```python
from build123d import *

# Parameters (mm, degrees)
F0_R     = 22.5
F1_DEPTH = 120
F3_DEPTH = 70
F4_R     = 20
F5_DEPTH = 35
F6_R     = 2.5
F7_DEPTH = 50


with BuildPart() as f1:
    # F0 (on Top) → F1 (new body)
    with BuildSketch(Plane.XY):
        Circle(F0_R)
    extrude(amount=F1_DEPTH)

    # F2 (on face) → F3 (cut)
    with BuildSketch(Plane.XY.offset(120)):
        with BuildLine():
            ThreePointArc((22.5, 0), (19.843135, 10.606602), (12.5, 18.708287))
            Line((12.5, 18.708287), (12.5, -18.708287))
            ThreePointArc((12.5, -18.708287), (19.843135, -10.606602), (22.5, 0))
        make_face()
        with BuildLine():
            Line((-12.5, -18.708287), (-12.5, 18.708287))
            ThreePointArc((-12.5, 18.708287), (-22.5, 0), (-12.5, -18.708287))
        make_face()
    extrude(amount=-F3_DEPTH, mode=Mode.SUBTRACT)

    # F4 (on Top) → F5 (cut)
    with BuildSketch(Plane.XY):
        Circle(F4_R)
    extrude(amount=F5_DEPTH, mode=Mode.SUBTRACT)

    # F6 (on Right) → F7 (cut, symmetric)
    with BuildSketch(Plane.YZ):
        with Locations((0, 100)):
            Circle(F6_R)
    extrude(amount=F7_DEPTH, both=True, mode=Mode.SUBTRACT)


solid = f1.part
```
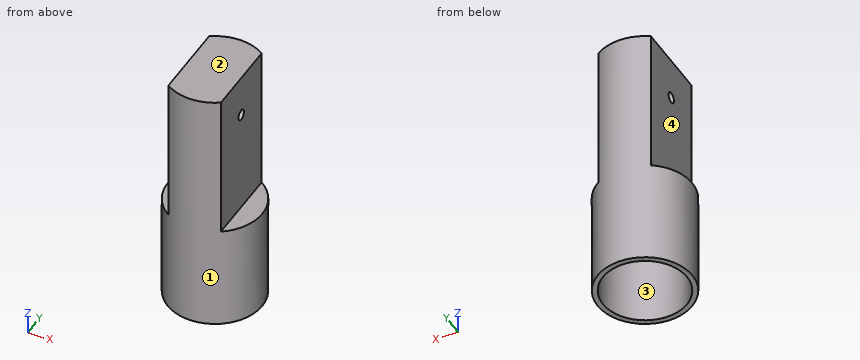
Check sheet for the modelled part. Datum: model origin and axes. Units: mm. Face numbers are marked on the shaded views. Coordinates: 2 decimals unless noted, no trailing zeros. Order: outer loops, then holes, each group sorted by start corner. A loop starts at its lowest first (then second) coordinate and runs counter-clockwise, first axis right, second up. Notation, with made-up numbers: (-3.75, -33) -> (14.25, -33) arc R12 cw to (14.25, -17) -> close; hole circle Ø1 at (-8.75, 83). An arc over 180 degrees is marked (long way). Write each question's results on one line, items separated by ' | '. Start each with the question number.
1) Draft check along X on the marked faces 1, 2, 3 and 4. Enter one of: pulls with the +X half, pulls with the -X half, needs draft (parallel to the pull), parting line crosses it, or undercut.
2) Depth check by flat-ended pin: pin 1 (1 mm diameter, centred on x = 17.5, y = 9, fed in from +Z); pin 2 (11 mm diameter, centred on y = 1, z = 76, fed in from -X); pin 3 (1.5 mm diameter, centred on x = 6, z = 61.5, fed in from +Y); pin 4 (11 mm diameter, centred on x = 15.5, y = -1, fed in from +Z). Enter the tip coordinate at first touch or a pass-through.
3) Material ranges on line 1 along Y through (x, z) = (0, 12); line 2 along Z through (x, y) = (4, 0); line 3 along Z through (x, y) = (-10, -4.5), recorded low to high.
4) Section check D-D (y = 13). Enter the section's corners in (x, z), and give its area (3 significant figures).
5) Section check A-A (z = 100). Enter the section's corners in (x, y), and give its area (3 significant figures).
6) Section check C-C (x = -4). Enter the section's corners in (y, z), and give its area (3 significant figures).
7) Section check B-B (y = 0). Enter the section's corners in (x, z), and give its area (4 significant figures).
Checked values:
1) face 1: parting line crosses it | face 2: needs draft | face 3: undercut | face 4: pulls with the -X half
2) pin 1: z = 50 | pin 2: x = -12.5 | pin 3: y = 21.88 | pin 4: z = 120
3) line 1: -22.5 to -20, 20 to 22.5 | line 2: 35 to 97.5, 102.5 to 120 | line 3: 35 to 120
4) outline: (-18.36, 0) -> (-15.2, 0) -> (-15.2, 35) -> (15.2, 35) -> (15.2, 0) -> (18.36, 0) -> (18.36, 50) -> (12.5, 50) -> (12.5, 120) -> (-12.5, 120) -> (-12.5, 50) -> (-18.36, 50) -> close | area: 2,520 mm²
5) outline: (-12.5, -18.71) arc R22.5 ccw to (12.5, -18.71) -> (12.5, -2.5) -> (-12.5, -2.5) -> close; (-12.5, 2.5) -> (12.5, 2.5) -> (12.5, 18.71) arc R22.5 ccw to (-12.5, 18.71) -> close | area: 939 mm²
6) outline: (-22.14, 0) -> (-19.6, 0) -> (-19.6, 35) -> (19.6, 35) -> (19.6, 0) -> (22.14, 0) -> (22.14, 120) -> (-22.14, 120) -> close; hole circle Ø5 at (0, 100) | area: 3,920 mm²
7) outline: (-22.5, 0) -> (-20, 0) -> (-20, 35) -> (20, 35) -> (20, 0) -> (22.5, 0) -> (22.5, 50) -> (12.5, 50) -> (12.5, 97.5) -> (-12.5, 97.5) -> (-12.5, 50) -> (-22.5, 50) -> close; (-12.5, 102.5) -> (12.5, 102.5) -> (12.5, 120) -> (-12.5, 120) -> close | area: 2,475 mm²
